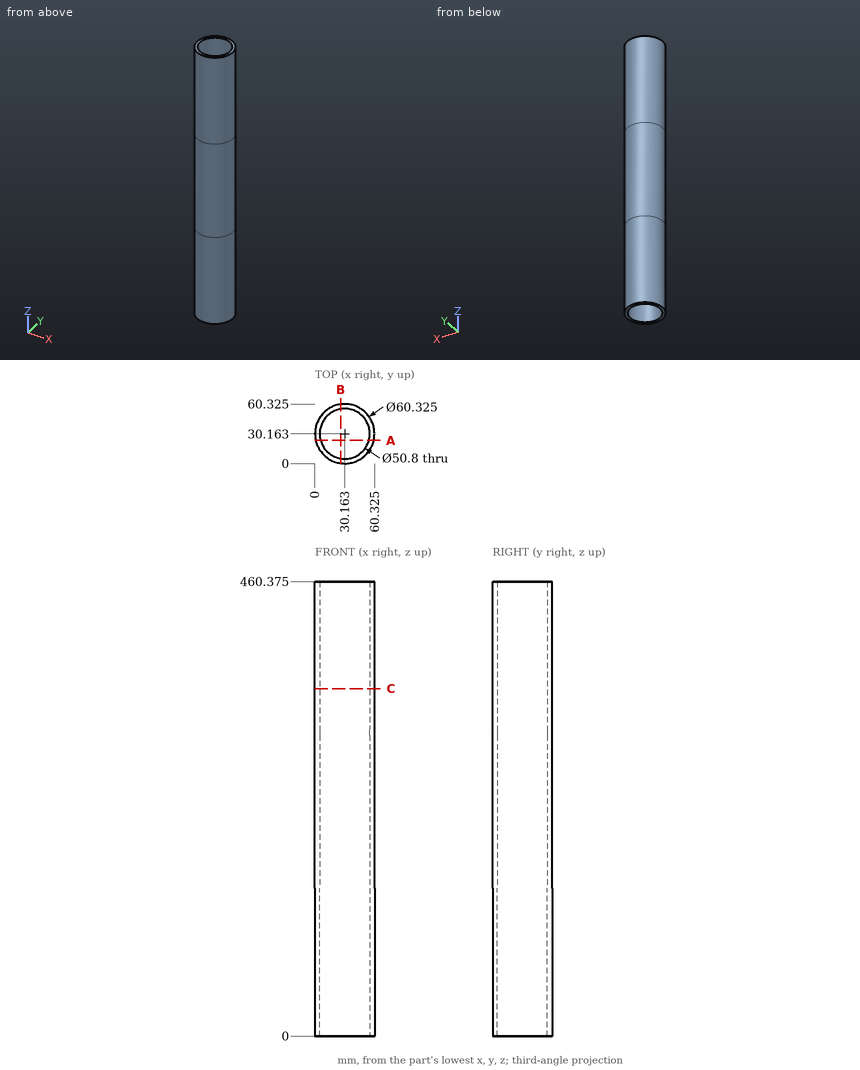
Could you check a few things on this drawing? It's one solid part, dimensions in mm from its lowest x, y, z. Give positions to 0.01 mm unless a question says otherwise; leave off trailing zeros. Order: outer loops, then holes, each group sorted by start corner. A loop starts at its lowest first (then second) coordinate and runs counter-clockwise, first axis right, second up. Notation, with made-up numbers: (-7.5, 82) - (51.5, 82) arc R30 ccw to (51.5, 116) - close; hole circle Ø10 at (43, 46.25). An arc over 180 degrees is marked (long way). One line per item, written item: value. Start each with the question number.
1. If I drill on probe 1 along X at (y, z) = (32, 98.5) (1 decimal); probe 2 along X at (y, z) = (30, 304.5) (1 decimal); probe 3 along Y at (x, z) = (44, 397.5) (1 decimal), over which ranges is the centre line in solid material (lowest first)?
2. For P1, Ø5, axis at x = 26, z = 110, coming from the +Y side; P2, Ø6, axis at x = 13.5, z = 370.5, coming from the +Y side; P3, Ø12, axis at y = 16, z = 186, coming from the +X side; P4, Ø4, axis at x = 53, y = 38.5, coming from the -Z side, each with a flat end and sliding along its axis, tell me the tip position at first contact or that it passes through.
3. Imagine slicing it at C-C on z = 352. List the corners of the cut face in (x, y) for me (1 decimal).
4. Imagine slicing it at A-A on y = 23.5. List the corners of the cut face in (x, z) for me (1 decimal).
5. Imagine slicing it at B-B on x = 26. List the corners of the cut face in (y, z) for me (1 decimal).
Values:
1. probe 1: 0.1 to 4.8, 55.5 to 60.3
1. probe 2: 0 to 4.8, 55.6 to 60.3
1. probe 3: 3.4 to 8.9, 51.5 to 57
2. P1: y = 60.28
2. P2: y = 57.05
2. P3: x = 59.2
2. P4: z = 0
3. outline: circle Ø60.3 at (30.2, 30.2); hole circle Ø50.8 at (30.2, 30.2)
4. outline: (0.7, 0) - (5.7, 0) - (5.7, 460.4) - (0.7, 460.4) - close; (54.7, 0) - (59.6, 0) - (59.6, 460.4) - (54.7, 460.4) - close
5. outline: (0.3, 0) - (5.1, 0) - (5.1, 460.4) - (0.3, 460.4) - close; (55.2, 0) - (60, 0) - (60, 460.4) - (55.2, 460.4) - close
